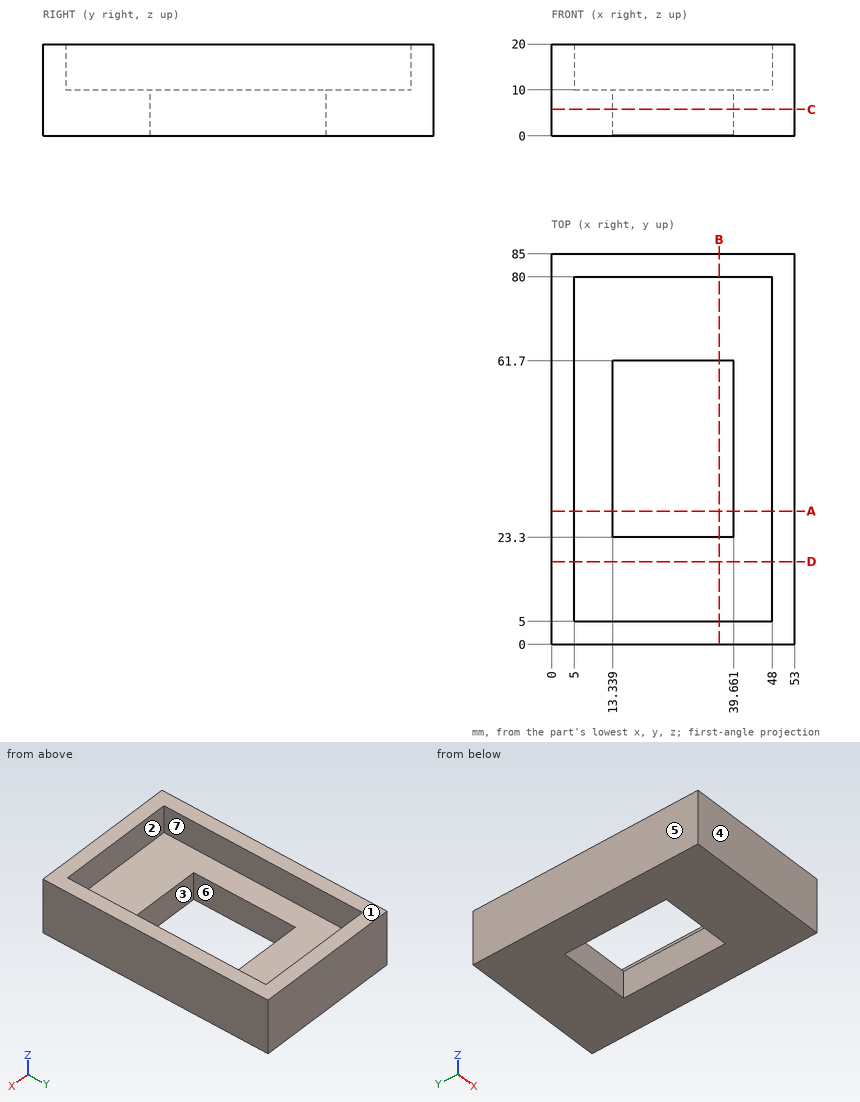
The figure shows three views and two pictorial views of one solid part (mm, origin at its lowest corner). Answer the questions. A direction names the side the tool comes from. Coordinates: 2 decimals unless noted, no trailing zeros. Loops run counter-clockwise (first coordinate to the right, second up) from the corner with the lowest first, then second, coordinate; pieces in that order, holes last. Notation, with made-up numbers: (-6.75, 12.25) -> (-2.75, 12.25) arc R29 ccw to (-2.75, 48.25) -> close; hole circle Ø10 at (-1, 49). An arc over 180 degrees is marked (long way). Return JSON: item names as keys, results as strings. Group by question number.
(1) Find the intervals of material crossed by probe 1 along Y at (x, z) = (24.5, 7.25); probe 2 along Y at (x, z) = (27.5, 13.5); probe 3 along X at (y, z) = (67, 14.75), in increasing order. Write a range as from..to.
(2) A cutting plane is placed at B-B on x = 36.5. Write down the section's boundary in (y, z).
(3) Which of the six approach directions +Z, -Z, +X, -X, +Y, -Y give full straight-line access (tool end or side, diameter ignored) to the marked faces 5, 6 and 7?
(4) Determine the mould class of the marked faces 1, 2, 3 and 4 for opening direction Y: released by +Y, released by -Y, zero draft, split by the parting line, or undercut.
(5) A cutting plane is placed at D-D on y = 18. Write down the section's boundary in (x, z), and give its area (3 significant figures).
(6) A cutting plane is placed at C-C on z = 5.75. Write down the section's boundary in (x, y), and give its area (3 significant figures).
(7) A cutting plane is placed at A-A on y = 29. Write down the section's boundary in (x, z).
The answers:
{
 "1": {"probe 1": "y = 0..23.3, 61.7..85", "probe 2": "y = 0..5, 80..85", "probe 3": "x = 0..5, 48..53"},
 "2": {"outline": "(0, 0) -> (23.3, 0) -> (23.3, 10) -> (5, 10) -> (5, 20) -> (0, 20) -> close; (61.7, 0) -> (85, 0) -> (85, 20) -> (80, 20) -> (80, 10) -> (61.7, 10) -> close"},
 "3": {"face 5": "+Z, -Z, -X, +Y, -Y", "face 6": "+Z, -Z", "face 7": "+Z"},
 "4": {"face 1": "zero draft", "face 2": "undercut", "face 3": "undercut", "face 4": "released by -Y"},
 "5": {"outline": "(0, 0) -> (53, 0) -> (53, 20) -> (48, 20) -> (48, 10) -> (5, 10) -> (5, 20) -> (0, 20) -> close", "area": "630 mm^2"},
 "6": {"outline": "(0, 0) -> (53, 0) -> (53, 85) -> (0, 85) -> close; hole (13.34, 23.3) -> (39.66, 23.3) -> (39.66, 61.7) -> (13.34, 61.7) -> close", "area": "3,490 mm^2"},
 "7": {"outline": "(0, 0) -> (13.34, 0) -> (13.34, 10) -> (5, 10) -> (5, 20) -> (0, 20) -> close; (39.66, 0) -> (53, 0) -> (53, 20) -> (48, 20) -> (48, 10) -> (39.66, 10) -> close"}
}
